```python
from build123d import *

# Parameters (mm, degrees)
F1_DEPTH = 63.5
F0_W     = 26.390754
F0_H     = 19.05
F2_DEPTH = 25.4
F3_DEPTH = 19.05


with BuildPart() as f1:
    # F0 (on Front) → F1 (new body, symmetric)
    with BuildSketch(Plane.XZ):
        Polygon((22.225, 9.525), (-41.275, 9.525), (-41.275, -9.525), (41.275, -9.525), (41.275, 9.525), align=None)
    extrude(amount=F1_DEPTH, both=True)

    # F0 (on Front) → F2 (join, symmetric)
    with BuildSketch(Plane.XZ):
        with BuildLine():
            Line((22.225, 28.575), (22.225, 9.525))
            Line((22.225, 9.525), (41.275, 9.525))
            Line((41.275, 9.525), (41.275, 28.575))
            ThreePointArc((41.275, 28.575), (45.92468, 39.80032), (57.15, 44.45))
            Line((57.15, 44.45), (62.56327, 44.45))
            Line((62.56327, 44.45), (62.56327, 63.5))
            Line((62.56327, 63.5), (57.15, 63.5))
            add(Edge.make_bspline(
                [(50.745571, 62.907767), (52.916409, 63.149474), (55.054315, 63.3464), (57.15, 63.5)],
                knots=[105.739127, 105.739127, 105.739127, 105.739127, 112.253202, 112.253202, 112.253202, 112.253202], degree=3))
            ThreePointArc((50.745571, 62.907767), (30.285243, 50.891821), (22.225, 28.575))
        make_face()
        with Locations((75.758647, 53.975)):
            Rectangle(F0_W, F0_H)
    extrude(amount=F2_DEPTH, both=True)

    # F0 (on Front) → F3 (join, symmetric)
    with BuildSketch(Plane.XZ):
        with BuildLine():
            add(Edge.make_bspline(
                [(-41.275, 9.525), (-28.407678, 43.261675), (15.507642, 58.984288), (50.745571, 62.907767)],
                knots=[0, 0, 0, 0, 105.739127, 105.739127, 105.739127, 105.739127], degree=3))
            Line((-41.275, 9.525), (22.225, 9.525))
            Line((22.225, 9.525), (22.225, 28.575))
            ThreePointArc((22.225, 28.575), (30.285243, 50.891821), (50.745571, 62.907767))
        make_face()
    extrude(amount=F3_DEPTH, both=True)


solid = f1.part
```
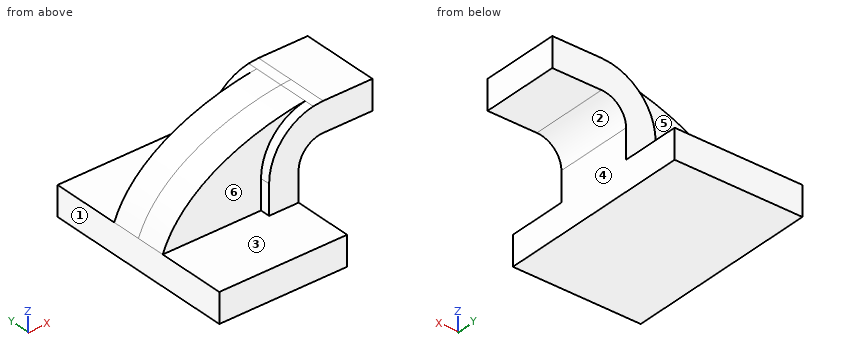
Input: part model. Units: mm. Frame: model coordinates. Face numbers are marked on the shaded views. A direction names the side the tool comes from. Coordinates: 2 decimals unless noted, no trailing zeros. Loops run counter-clockwise (first coordinate to the right, second up) from the corner with the lowest first, then second, coordinate; pieces in that order, holes last. Notation, with made-up numbers: M -27,52.5 L 32,52.5 A21 cw 32,64.5 Z; hole C -12,3.5 d8. An arc over 180 degrees is marked long. Answer in a Markdown table with one row per item.
1. Section B-B, the plane z = 5. Output: boundary loops of the cut face in (x, y) (3 decimals).
Response:
| item | result |
|---|---|
| outline | M -41.275,-63.5 L 41.275,-63.5 L 41.275,63.5 L -41.275,63.5 Z |
2. First-contact query: pin 1 (1.5 mm diameter, centred on y = -1.5, z = 30.5, fed in from -X); pin 2 (4 mm diameter, centred on y = 12, z = 48.5, fed in from -X); pin 3 (19 mm diameter, centred on y = -9, z = 15.5, fed in from +X) (3 decimals). Flat tips, straight axial feed; report the tip coordinate or a pass-through.
Response:
| item | result |
|---|---|
| pin 1 | stops at x = -28.21 |
| pin 2 | stops at x = -5.38 |
| pin 3 | stops at x = 41.275 |
3. Section A-A, the plane x = 70.5. Output: boundary loops of the cut face in (y, z).
Response:
| item | result |
|---|---|
| outline | M -25.4,44.45 L 25.4,44.45 L 25.4,63.5 L -25.4,63.5 Z |
4. Draft query along X for the marked faces 1, 2 and 3. Return one class per face: pulls with the +X half, pulls with the -X half, needs draft (parallel to the pull), parting line crosses it, or undercut.
Response:
| item | result |
|---|---|
| face 1 | pulls with the -X half |
| face 2 | pulls with the +X half |
| face 3 | needs draft |
5. Material intervals for line 1 (Z direction, x = -5.5, y = 46.5) (3 decimals); line 2 (Z direction, x = 77, y = 16.5); line 3 (Y direction, x = -12, z = 20), sorted ascending.
Response:
| item | result |
|---|---|
| line 1 | z = -9.525 to 9.525 |
| line 2 | z = 44.45 to 63.5 |
| line 3 | y = -19.05 to 19.05 |
6. Reachability of the marked faces 4, 5 and 6 from +Z, -Z, +X, -X, +Y, -Y: full face, straight path, thin tool, end or side. Return the list, or none.
Response:
| item | result |
|---|---|
| face 4 | -Z, +X, +Y, -Y |
| face 5 | +Z, -X, +Y |
| face 6 | +Z, -X, -Y |
